CAD build for the part. Positions are in the model's coordinates, mm. A direction names the side the tool comes from. Coordinates: 2 decimals unless noted, no trailing zeros. Loops run counter-clockwise (first coordinate to the right, second up) from the corner with the lowest first, then second, coordinate; pieces in that order, holes last. Notation, with made-up numbers: (59, -39) -> (110, -39) arc R28 cw to (110, -20) -> close; hole circle Ø5 at (37.5, -10). An arc over 180 degrees is marked (long way). Write each question's results on one line, items separated by ' | '.
```python
from build123d import *

# Parameters (mm, degrees)
F1_DEPTH = 1.27
F2_R     = 0.817287
F3_DEPTH = 12.7


with BuildPart() as f1:
    # F0 (on Top) → F1 (new body)
    with BuildSketch(Plane.XY):
        Polygon((2.120686, -2.821234), (0, -2.821234), (0, -25.078306), (16.910204, -22.496327), align=None)
        Polygon((-1.991502, 2.649376), (0, 2.649376), (0, 21.549277), (-16.198318, 21.549277), align=None)
        Polygon((0, 21.549277), (0, 2.649376), (1.909298, 2.649376), (15.529687, 21.549277), align=None)
        Polygon((24.537329, 0), (2.733955, 0), (2.733955, -1.97025), (22.622143, -16.302859), align=None)
        Polygon((2.733955, 2.055079), (2.733955, 0), (24.537329, 0), (21.880006, 16.446924), align=None)
        Polygon((-25.219401, 0), (-2.87027, 0), (-2.87027, 2.068487), (-22.82205, 16.446924), align=None)
        Polygon((-2.87027, -2.157545), (-2.87027, 0), (-25.219401, 0), (-22.667898, -17.039172), align=None)
        Polygon((0, -25.078306), (0, -2.821234), (-2.033148, -2.821234), (-16.454118, -22.832033), align=None)
        Polygon((2.733955, 0), (0, 0), (0, -2.821234), (2.120686, -2.821234), (2.733955, -1.97025), align=None)
        Polygon((0, 2.649376), (0, 0), (2.733955, 0), (2.733955, 2.055079), (1.909298, 2.649376), align=None)
        Polygon((-2.87027, 0), (0, 0), (0, 2.649376), (-1.991502, 2.649376), (-2.87027, 2.068487), align=None)
        Polygon((0, -2.821234), (0, 0), (-2.87027, 0), (-2.87027, -2.157545), (-2.033148, -2.821234), align=None)
    extrude(amount=F1_DEPTH)

    # F2 (on face) → F3 (cut)
    with BuildSketch(Plane.XY.offset(1.27)):
        with Locations((0, 20.010149)):
            Circle(F2_R)
    extrude(amount=-F3_DEPTH, mode=Mode.SUBTRACT)


solid = f1.part
```
Q1. Cut at B-B on z = 0.35. Write the cut outline in (x, y), and give its area (3 significant figures).
Results are:
outline: (-25.22, 0) -> (-22.67, -17.04) -> (-2.87, -2.16) -> (-2.03, -2.82) -> (-16.45, -22.83) -> (0, -25.08) -> (16.91, -22.5) -> (2.12, -2.82) -> (2.73, -1.97) -> (22.62, -16.3) -> (24.54, 0) -> (21.88, 16.45) -> (2.73, 2.06) -> (1.91, 2.65) -> (15.53, 21.55) -> (-16.2, 21.55) -> (-1.99, 2.65) -> (-2.87, 2.07) -> (-22.82, 16.45) -> close; hole circle Ø1.63 at (0, 20.01) | area: 1,590 mm^2
Q2. Pull direction X, two halves, no side cores. Call faces 3 (the flat face through (-12.71, 9.16, 0.63)), 4 (the flat face through (-1, -1, 0)), 5 (the flat face through (-24.004, 8.339, 0.626)): +X half, -X half, draft (parallel to the pull), parting line (faces both ways), or undercut.
Results are:
face 3: undercut | face 4: draft | face 5: -X half
Q3. Cut at C-C on y = -6. Write the cut outline in (x, z).
Results are:
outline: (-24.32, 0) -> (-7.98, 0) -> (-7.98, 1.27) -> (-24.32, 1.27) -> close; (-4.32, 0) -> (4.51, 0) -> (4.51, 1.27) -> (-4.32, 1.27) -> close; (8.33, 0) -> (23.83, 0) -> (23.83, 1.27) -> (8.33, 1.27) -> close
Q4. Drop a flat-ended pin along its axis: pin 1 (1.9 mm diameter, centred on x = 0, y = 20.01, fed in from -Z). Give the stop position or say it passes through.
Results are:
pin 1: z = 0
Q5. Cut at A-A on y = 8. Write the cut outline in (x, z), and give its area (3 significant figures).
Results are:
outline: (-24.05, 0) -> (-11.1, 0) -> (-11.1, 1.27) -> (-24.05, 1.27) -> close; (-6.01, 0) -> (5.77, 0) -> (5.77, 1.27) -> (-6.01, 1.27) -> close; (10.64, 0) -> (23.24, 0) -> (23.24, 1.27) -> (10.64, 1.27) -> close | area: 47.4 mm^2
Q6. Which spindle directions (+Z, -Z, +X, -X, +Y, -Y) get a long thin tool onto all of the face, cutting with end or side? Do faces 1 (the flat face through (23.566, -8.266, 0.626)), 2 (the flat face through (12.539, -9.036, 0.626)). Say none if no direction does.
Results are:
face 1: +Z, -Z, +X, -Y | face 2: +Z, -Z
Q7. Wall check: L1, parallel to X at y = 15, z = 1; L2, parallel to X at y = -4, z = 0.1; L3, parallel to Y at x = 0, z = 0.2. Give the ranges that are in metal, low to high. Write a range as from..to.
Results are:
L1: -23.03..-20.81, -11.28..10.81, 19.96..22.11 | L2: -24.62..-5.32, -2.88..3.01, 5.55..24.07 | L3: -25.08..19.19, 20.83..21.55
